Autodesk Inventor part; units mm, degrees
ref_plane "YZ Plane" through (0, 0, 0) normal (1, 0, 0) x (0, 1, 0)
ref_plane "XZ Plane" through (0, 0, 0) normal (0, 1, 0) x (-1, 0, 0)
ref_plane "XY Plane" through (0, 0, 0) normal (0, 0, 1) x (1, 0, 0)
sketch "Sketch1" plane through (0, 0, 0) normal (0, 1, 0) x (-1, 0, 0)
  line L0 (18, 35) -> (-12, 35)
  line L1 (-12, 35) -> (-12, -35)
  line L2 (-12, -35) -> (18, -35)
  line L3 (18, -35) -> (18, 35)
  circle A0 centre (0, 0) radius 2.5
  circle A1 centre (0, -25) radius 2.5
  circle A2 centre (0, 25) radius 2.5
  dimension "d0" = 5
  dimension "d1" = 25
  dimension "d2" = 25
  dimension "d3" = 10
  dimension "d4" = 10
  dimension "d5" = 30
  dimension "d6" = 12
extrude "Extrusion1" add sketch "Sketch1" along normal blind 3
properties part number "testing_chunk"
Geometry check sheet. Reference: the model listing, model coordinates, mm. Round coordinates to 2 decimals unless told otherwise and drop trailing zeros. Write each loop counter-clockwise with the first axis right and the second up, starting at its lowest first coordinate (ties: lowest second). Pieces come first, ordered by that corner, then holes. Notation, with made-up numbers: (53, -9) -> (59, -9) arc R12 cw to (59, 5) -> close; hole circle Ø5 at (44, 23). An arc over 180 degrees is marked (long way). One line per item, written item: value. Start each with the question number.
(1) Scan lines: line 1 (Z direction, x = 0, y = 1.6); line 2 (Z direction, x = -1.25, y = 0.35); line 3 (X direction, y = 2.55, z = 23). Record each from-to range of solid material in increasing order. Write a range as [from, to].
(2) Cross-section at D-D, the plane z = 0. Record the cut outline in (x, y).
(3) Go/stop test with a flat-tipped pin: pin 1 Ø3 at (x, z) = (0, 25) entering from +Y. Record where the tip stops, or that it passes through.
(4) Cross-section at C-C, the plane y = 1.05. Record the cut outline in (x, z), and give its area (3 significant figures).
(5) Cross-section at B-B, the plane x = 0. Record the cut outline in (y, z).
(6) Draft check along Z on faces 1 (the cylindrical face through (0.33, 1.48, 22.52)), 2 (the flat face through (-3, 0, 0)), 3 (the flat face through (-3, 1, 35)). Enter one of: +Z half, -Z half, draft (parallel to the pull), parting line (faces both ways), or undercut.
(7) Cross-section at A-A, the plane z = 23.5. Record the cut outline in (x, y).
Answer:
1. line 1: [-35, -27.5], [-22.5, -2.5], [2.5, 22.5], [27.5, 35]
1. line 2: [-35, -27.17], [-22.83, -2.17], [2.17, 22.83], [27.17, 35]
1. line 3: [-18, -1.5], [1.5, 12]
2. outline: (-18, 0) -> (-2.5, 0) -> (-2.5, 3) -> (-18, 3) -> close; (2.5, 0) -> (12, 0) -> (12, 3) -> (2.5, 3) -> close
3. pin 1: through
4. outline: (-18, -35) -> (12, -35) -> (12, 35) -> (-18, 35) -> close; hole circle Ø5 at (0, -25); hole circle Ø5 at (0, 0); hole circle Ø5 at (0, 25)
4. area: 2,040 mm²
5. outline: (0, -35) -> (3, -35) -> (3, -27.5) -> (0, -27.5) -> close; (0, -22.5) -> (3, -22.5) -> (3, -2.5) -> (0, -2.5) -> close; (0, 2.5) -> (3, 2.5) -> (3, 22.5) -> (0, 22.5) -> close; (0, 27.5) -> (3, 27.5) -> (3, 35) -> (0, 35) -> close
6. face 1: undercut
6. face 2: draft
6. face 3: +Z half
7. outline: (-18, 0) -> (-2, 0) -> (-2, 3) -> (-18, 3) -> close; (2, 0) -> (12, 0) -> (12, 3) -> (2, 3) -> close
